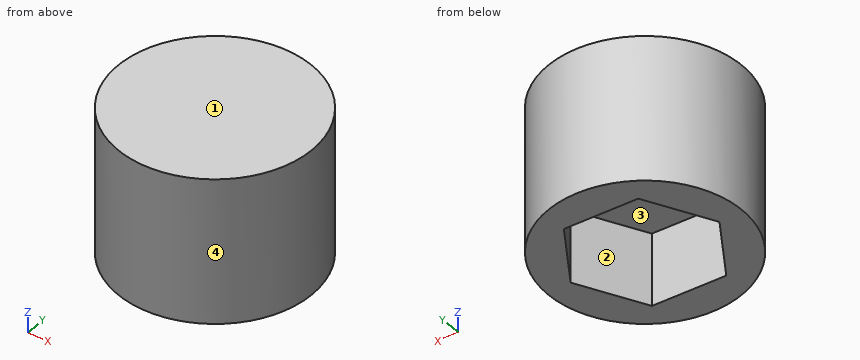
```python
from build123d import *

# Parameters (mm, degrees)
SKETCH_1_R          = 4
EXTRUDE_1_DEPTH     = 6
CUT_EXTRUDE_1_DEPTH = 3


with BuildPart() as part:
    # 草图1 → 凸台-拉伸1 (new body)
    with BuildSketch(Plane.XY):
        Circle(SKETCH_1_R)
    extrude(amount=EXTRUDE_1_DEPTH)

    # 草图3 → 切除-拉伸1 (cut)
    with BuildSketch(Plane(origin=(0, 0, 0), x_dir=(-1, 0, 0), z_dir=(0, 0, -1))):
        Polygon((2.998599074, -0.091671127), (1.578689062, 2.55102741), (-1.419910012, 2.642698537), (-2.998599074, 0.091671127), (-1.578689062, -2.55102741), (1.419910012, -2.642698537), align=None)
    extrude(amount=-CUT_EXTRUDE_1_DEPTH, mode=Mode.SUBTRACT)


solid = part.part
```
Input: part model. Units: mm. Frame: model coordinates. Face numbers are marked on the shaded views. Round coordinates to 2 decimals unless told otherwise and drop trailing zeros. Loops run counter-clockwise (first coordinate to the right, second up) from the corner with the lowest first, then second, coordinate; pieces in that order, holes last. Notation, with made-up numbers: M 69,54 L 116,54 A12 cw 116,59 Z; hole C 78,-20.5 d10. An arc over 180 degrees is marked long. Answer in a Markdown table with one row per item. Add a question column.
1. Section C-C (x = -1.25). Output: boundary loops of the cut face in (y, z), and give its area (3 significant figures).
2. Section D-D (z = 3.4). Output: boundary loops of the cut face in (x, y).
3. Mould query, pull axis Y, two halves, no side actions, for the marked faces 1, 2, 3 and 4. Classes: released by +Y, released by -Y, zero draft, split by the parting line, or undercut.
4. Section B-B (y = 0.75). Output: boundary loops of the cut face in (x, z), and give its area (3 significant figures).
5. Ray query, probe 1 along Z at (x, y) = (1.25, -0.5); probe 2 along X at (y, z) = (-1.25, 2.8); probe 3 along Y at (x, z) = (-2.75, 1). Return the intervals inside material, ascending.
6. Contact query for a flat-ended pin moving along its axis: pin 1 (1 mm diameter, centred on x = 2.5, z = 1.5, fed in from +Y). Output: stop coordinate, or through.
7. Section A-A (z = 1.25). Output: boundary loops of the cut face in (x, y), and give its area (3 significant figures).
Values follow:
| question | item | result |
|---|---|---|
| 1 | outline | M -3.8,0 L -2.64,0 L -2.64,3 L 2.56,3 L 2.56,0 L 3.8,0 L 3.8,6 L -3.8,6 Z |
| 1 | area | 30.0 mm^2 |
| 2 | outline | C 0,0 d8 |
| 3 | face 1 | zero draft |
| 3 | face 2 | undercut |
| 3 | face 3 | undercut |
| 3 | face 4 | split by the parting line |
| 4 | outline | M -3.93,0 L -2.55,0 L -2.55,3 L 2.59,3 L 2.59,0 L 3.93,0 L 3.93,6 L -3.93,6 Z |
| 4 | area | 31.7 mm^2 |
| 5 | probe 1 | 3 to 6 |
| 5 | probe 2 | -3.8 to -2.28, 2.28 to 3.8 |
| 5 | probe 3 | -2.9 to -0.49, 0.37 to 2.9 |
| 6 | pin 1 | y = 3.46 |
| 7 | outline | C 0,0 d8; hole M -3,-0.09 L -1.42,-2.64 L 1.58,-2.55 L 3,0.09 L 1.42,2.64 L -1.58,2.55 Z |
| 7 | area | 26.9 mm^2 |
